Autodesk Inventor part; units mm, degrees
ref_plane "YZ Plane" through (0, 0, 0) normal (1, 0, 0) x (0, 1, 0)
ref_plane "XZ Plane" through (0, 0, 0) normal (0, 1, 0) x (-1, 0, 0)
ref_plane "XY Plane" through (0, 0, 0) normal (0, 0, 1) x (1, 0, 0)
sketch "Szkic1" plane through (0, 0, 0) normal (0, 0, 1) x (1, 0, 0)
  circle A0 centre (0, 0) radius 50
  line L0 (-25, 25) -> (-12.5, 25)
  line L1 (-12.5, -25) -> (-25, -25)
  line L2 (-25, -25) -> (-25, 25)
  line L3 (-12.5, -25) -> (-12.5, 25)
  point P0 (-12.5, 0)
  point P1 (-18.75, 25)
  dimension "d0" = 100
  dimension "d10" = 12.5
  dimension "d11" = 12.5
  dimension "d12" = 50
  dimension "d13" = 25
extrude "Wyciągnięcie proste1" add sketch "Szkic1" along normal blind 60 contours L0 L3 L1 L2
extrude "Wyciągnięcie proste2" add sketch "Szkic1" along normal blind 10 contours A0 | L0 L3 L1 L2
sketch "Szkic2" plane through (-25, -25, 60) normal (-1, 0, 0) x (0, 0, 1)
  line L0 (-50, 50) -> (-50, 0)
  line L1 (-50, 0) -> (0, 0)
  line L2 (0, 50) -> (0, 0)
  line L3 (-50, 50) -> (0, 50)
  circle A0 centre (-25, 25) radius 25
  line L4 (-50, 50) -> (0, 50)
  line L5 (0, 50) -> (0, 0)
  line L6 (-25, 50) -> (0, 50)
  line L7 (0, 25) -> (0, 0)
  point P0 (-60, 25)
  point P1 (-25, 50)
  point P2 (0, 25)
  point P3 (-25, 0)
  dimension "d7" = 50
extrude "Wyciągnięcie proste3" cut sketch "Szkic2" against normal through all contours L3 L2 A0 | A0 L2 L1
properties part number "podstawa"
Part model, mm, in its own coordinate system. A direction names the side the tool comes from. Give positions to 0.01 mm unless a question says otherwise; leave off trailing zeros. Write each loop counter-clockwise with the first axis right and the second up, starting at its lowest first coordinate (ties: lowest second). Pieces come first, ordered by that corner, then holes.
1) Cut at A-A on y = 0. Write the cut outline in (x, z), then the cut area to 4 significant figures.
Resolved:
outline: (-50, 0) - (50, 0) - (50, 10) - (-12.5, 10) - (-12.5, 60) - (-25, 60) - (-25, 10) - (-50, 10) - close
area: 1,625 mm2
2) Probe L1, parallel to Z at x = 38, y = -21.5; L2, parallel to X at y = -15.5, z = 12; L3, parallel to Z at x = -19.5, y = 18.5. List the from-to ranges inside material, lowest first.
Resolved:
L1: z = 0 to 10
L2: x = -25 to -12.5
L3: z = 0 to 51.82
3) Cut at C-C on x = 0. Write the cut outline in (y, z), then the cut area to 3 significant figures.
Resolved:
outline: (-50, 0) - (50, 0) - (50, 10) - (-50, 10) - close
area: 1,000 mm2
4) Cut at B-B on z = 42. Write the cut outline in (x, y).
Resolved:
outline: (-25, -24) - (-12.5, -24) - (-12.5, 24) - (-25, 24) - close
5) Which spindle directions (+Z, -Z, +X, -X, +Y, -Y) get a long thin tool onto all of the face, cutting with end or side? Do faces 1 (the face through (-19, -25, 22)), 2 (the face through (-19, 25, 22)), 3 (the face through (-25, 0, 35)). Say none if no direction does.
Resolved:
face 1: +Z, +X, -X, -Y
face 2: +Z, +X, -X, +Y
face 3: +Z, -X, +Y, -Y
6) Pin check, flat tips, straight feed: pin 1 (14 mm diameter, centred on x = -20.5, z = 20, fed in from -Y); pin 2 (10 mm diameter, centred on y = -13.5, z = 38, fed in from +X); pin 3 (4 mm diameter, centred on x = -22, z = 14.5, fed in from +Y); pin 4 (2 mm diameter, centred on y = -27, z = 19, fed in from +X). Stop position of each tip, or through.
Resolved:
pin 1: stops at y = -25
pin 2: stops at x = -12.5
pin 3: stops at y = 25
pin 4: passes through
7) Cut at D-D on y = -17.5. Write the cut outline in (x, z), then the cut area to 3 significant figures.
Resolved:
outline: (-46.84, 0) - (46.84, 0) - (46.84, 10) - (-12.5, 10) - (-12.5, 52.85) - (-25, 52.85) - (-25, 10) - (-46.84, 10) - close
area: 1,470 mm2
